The listing builds one solid part. Answer for the finished solid, in the listing's coordinates (mm). Face numbers are marked on the shaded views. A direction names the side the tool comes from. Round coordinates to 2 decimals unless told otherwise and drop trailing zeros. Write each loop counter-clockwise with the first axis right and the second up, starting at its lowest first coordinate (ties: lowest second). Pieces come first, ordered by that corner, then holes.
(1) Each of these flat-tipped pins is pushed along its axis until it touches: pin 1 Ø3.5 at (y, z) = (9, 0) entering from -X (3 decimals); pin 2 Ø1.9 at (x, z) = (-38.5, 2) entering from -Y; pin 3 Ø4 at (x, z) = (-50.3, -15.3) entering from +Y. Where does it stop, or does it pass through?
(2) A cutting plane is placed at D-D, the plane z = -5. Give the vertices of the cut face in (x, y) (3 decimals), and give its area (3 significant figures).
(3) A cutting plane is placed at A-A, the plane y = 9.75. Give the vertices of the cut face in (x, z) (3 decimals).
(4) Find the intervals of material crossed by probe 1 along X at (y, z) = (0.45, -66.1); probe 2 along Z at (x, y) = (-7.2, 0.5); probe 3 along X at (y, z) = (7.5, 2) (3 decimals), in increasing order.
(5) A cutting plane is placed at B-B, the plane z = -66.1. Give the vertices of the cut face in (x, y), and give its area (3 significant figures).
(6) For the marked faces 5, 6 and 7, determine the directions among +Z, -Z, +X, -X, +Y, -Y from which every point of the face is accessible in a straight line to the end or side of a thin tool.
(7) A cutting plane is placed at C-C, the plane x = -35.1. Give the vertices of the cut face in (y, z) (3 decimals).
(8) The mould has two halves that part along X. Classify the marked faces 1, 2, 3 and 4: +X half, -X half, draft (parallel to the pull), parting line (faces both ways), or undercut.
Autodesk Inventor part; units mm, degrees
ref_plane "YZ Plane" through (0, 0, 0) normal (1, 0, 0) x (0, 1, 0)
ref_plane "XZ Plane" through (0, 0, 0) normal (0, 1, 0) x (-1, 0, 0)
ref_plane "XY Plane" through (0, 0, 0) normal (0, 0, 1) x (1, 0, 0)
sketch "Sketch1" plane through (0, 0, 0) normal (0, 1, 0) x (-1, 0, 0)
  line L0 (0, 0) -> (53.3, 0)
  line L1 (53.3, 0) -> (53.3, -68.6)
  line L2 (53.3, -68.6) -> (0, -68.6)
  line L3 (0, -68.6) -> (0, 0)
  dimension "d0" = 68.6
  dimension "d1" = 53.3
extrude "Extrusion1" add sketch "Sketch1" along normal blind 1.6
sketch "Sketch2" plane through (0, 1.6, 0) normal (0, 1, 0) x (1, 0, 0)
  circle A0 centre (-50.3, 15.3) radius 1.6
  circle A1 centre (-2.5, 14.2) radius 1.6
  circle A2 centre (-7.2, 66.1) radius 1.6
  circle A3 centre (-35.1, 66.1) radius 1.6
  line L0 (-53.3, 0) -> (0, 0)
  line L1 (0, 0) -> (0, 68.6)
  dimension "d5" = 3.2
  dimension "d6" = 51.9
  dimension "d7" = 50.8
  dimension "d8" = 27.9
  dimension "d9" = 15.2
  dimension "d10" = 4.7
  dimension "d11" = 15.3
  dimension "d12" = 2.5
extrude "Extrusion2" cut sketch "Sketch2" against normal through all
sketch "Sketch3" plane through (0, 1.6, 0) normal (0, 1, 0) x (1, 0, 0)
  line L0 (-43.775, 9.525) -> (-31.775, 9.525)
  line L1 (-31.775, 9.525) -> (-31.775, -6.2)
  line L2 (-31.775, -6.2) -> (-43.775, -6.2)
  line L3 (-43.775, -6.2) -> (-43.775, 9.525)
  line L4 (-12.2, 11.43) -> (-3.3, 11.43)
  line L5 (-3.3, 11.43) -> (-3.3, -6.2)
  line L6 (-3.3, -6.2) -> (-12.2, -6.2)
  line L7 (-12.2, -6.2) -> (-12.2, 11.43)
  line L8 (-53.3, 0) -> (0, 0)
  line L9 (0, 0) -> (0, 68.6)
  line L10 (-53.3, 68.6) -> (-53.3, 0)
  dimension "d15" = 12
  dimension "d16" = 6.2
  dimension "d18" = 8.9
  dimension "d19" = 3.3
  dimension "d20" = 9.525
  dimension "d21" = 11.43
  dimension "d22" = 9.525
extrude "Extrusion3" add sketch "Sketch3" along normal blind 10.9
properties part number "Arduino_Model"
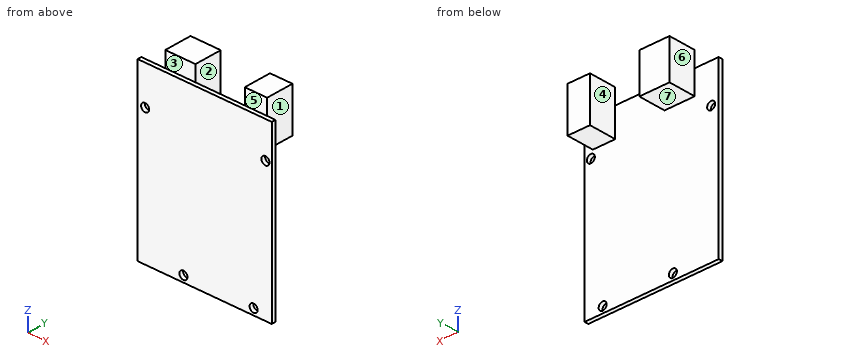
Solutions:
1. pin 1: stops at x = -43.775
1. pin 2: stops at y = 1.6
1. pin 3: stops at y = 1.6
2. outline: (-53.3, 0) - (0, 0) - (0, 1.6) - (-3.3, 1.6) - (-3.3, 12.5) - (-12.2, 12.5) - (-12.2, 1.6) - (-31.775, 1.6) - (-31.775, 12.5) - (-43.775, 12.5) - (-43.775, 1.6) - (-53.3, 1.6) - close
2. area: 313 mm2
3. outline: (-43.775, -9.525) - (-31.775, -9.525) - (-31.775, 6.2) - (-43.775, 6.2) - close; (-12.2, -11.43) - (-3.3, -11.43) - (-3.3, 6.2) - (-12.2, 6.2) - close
4. probe 1: x = -53.3 to -36.7, -33.5 to -8.8, -5.6 to 0
4. probe 2: z = -68.6 to -67.7, -64.5 to 0
4. probe 3: x = -43.775 to -31.775, -12.2 to -3.3
5. outline: (-53.3, 0) - (-36.7, 0) - (-36.7, 1.6) - (-53.3, 1.6) - close; (-33.5, 0) - (-8.8, 0) - (-8.8, 1.6) - (-33.5, 1.6) - close; (-5.6, 0) - (0, 0) - (0, 1.6) - (-5.6, 1.6) - close
5. area: 75.0 mm2
6. face 5: +Z, +X, -X, -Y
6. face 6: +Z, -Z, -X, +Y
6. face 7: -Z, -X, +Y
7. outline: (0, -68.6) - (1.6, -68.6) - (1.6, -67.7) - (0, -67.7) - close; (0, -64.5) - (1.6, -64.5) - (1.6, -9.525) - (12.5, -9.525) - (12.5, 6.2) - (1.6, 6.2) - (1.6, 0) - (0, 0) - close
8. face 1: +X half
8. face 2: undercut
8. face 3: draft
8. face 4: undercut
